For this review, take the finished solid that the model builds, in its own axes (mm). A direction names the side the tool comes from. Give positions to 0.01 mm unless a question says otherwise; leave off trailing zeros. Loops run counter-clockwise (first coordinate to the right, second up) from the corner with the lowest first, then second, coordinate; pieces in that order, holes last. Notation, with made-up numbers: (27.25, 60.25) - (68.25, 60.25) arc R23 cw to (68.25, 82.25) - close; hole circle Ø5 at (-2, -25). An arc over 180 degrees is marked (long way). Use CSV: the item, a comma, the result in double quotes. Start each with the question number.
1. Take a section at B-B on x = 0. Give the boundary of the cut face in (y, z).
2. For pin 1 (1.4 mm diameter, centred on y = 3, z = 13.5, fed in from -X); pin 2 (1.4 mm diameter, centred on y = 2.5, z = -13.5, fed in from +X), all flat-tipped, find the tip position at first contact; note any pin that passes through.
3. Take a section at C-C on z = 0. Give the boundary of the cut face in (x, y), plus the area to 3 significant figures.
4. For faces 1 (the flat face through (-4, 2, 13)), 2 (the cylindrical face through (6.59, 2.254, 11.495)), 3 (the flat face through (9.497, 2.318, -10.102)), 4 (the flat face through (-13.51, 2.32, 3.18)), list the 3-axis set-ups (+Z, -Z, +X, -X, +Y, -Y) from which the entire face can be reached by the end or side of a thin tool; tool diameter is ignored.
5. Wall thickness on line 1 (Z direction, x = 0, y = 3.6); line 2 (X direction, y = 1.9, z = 0); line 3 (Z direction, x = -8.5, y = 2.7): over which ranges is each line inside the solid? List them lowest first.
6. Mouldability with a two-part tool opening along Z and no side actions: class faces 5 (the cylindrical face through (-6.59, 2.254, -11.495)), 6 (the flat face through (-13.497, 2.318, -3.174)), 7 (the flat face through (-4, 2, -13)) as pulls with the +Z half, pulls with the -Z half, needs draft (parallel to the pull), parting line crosses it, or undercut.
7. Take a section at A-A on y = 3.75. Give the boundary of the cut face in (x, z).
```python
from build123d import *

# Parameters (mm, degrees)
SKETCH1_R           = 13.25
SKETCH1_R_2         = 10
BOSS_EXTRUDE1_DEPTH = 4.572
BOSS_EXTRUDE2_DEPTH = 4.572
CIRPATTERN1_COUNT   = 6


with BuildPart() as part:
    # Sketch1 → Boss-Extrude1 (new body)
    with BuildSketch(Plane(origin=(0, 0, 0), x_dir=(1, 0, 0), z_dir=(0, 1, 0))):
        Circle(SKETCH1_R)
        Circle(SKETCH1_R_2, mode=Mode.SUBTRACT)
    extrude(amount=BOSS_EXTRUDE1_DEPTH)

    # Sketch2 → Boss-Extrude2 (add)
    with BuildSketch(Plane(origin=(0, 4.572, 0), x_dir=(1, 0, 0), z_dir=(0, 1, 0))):
        with BuildLine():
            Line((-4, 12.631805097), (-4, 13.937359865))
            ThreePointArc((-4, 13.937359865), (0, 14.5), (4, 13.937359865))
            Line((4, 13.937359865), (4, 12.631805097))
            ThreePointArc((4, 12.631805097), (0, 13.25), (-4, 12.631805097))
        make_face()
    boss_extrude2 = extrude(amount=-BOSS_EXTRUDE2_DEPTH)

    # CirPattern1: Boss-Extrude2 ×6 about axis
    cirpattern1_axis = Axis((0, 0, 0), (0, 1, 0))
    for i in range(1, CIRPATTERN1_COUNT):
        add(boss_extrude2.rotate(cirpattern1_axis, i * 360 / CIRPATTERN1_COUNT))


solid = part.part
```
Check result:
1,outline,"(0, -14.5) - (4.57, -14.5) - (4.57, -10) - (0, -10) - close; (0, 10) - (4.57, 10) - (4.57, 14.5) - (0, 14.5) - close"
2,pin 1,"stops at x = -4"
2,pin 2,"stops at x = 4"
3,outline,"(-13.25, 0) - (-10, 0) - (-10, 4.57) - (-13.25, 4.57) - close; (10, 0) - (13.25, 0) - (13.25, 4.57) - (10, 4.57) - close"
3,area,"29.7 mm²"
4,face 1,"+Z, -X, +Y, -Y"
4,face 2,"+Z, +Y, -Y"
4,face 3,"-Z, +Y, -Y"
4,face 4,"-X, +Y, -Y"
5,line 1,"z = -14.5 to -10, 10 to 14.5"
5,line 2,"x = -13.25 to -10, 10 to 13.25"
5,line 3,"z = -10.16 to -5.27, 5.27 to 10.16"
6,face 5,"pulls with the -Z half"
6,face 6,"undercut"
6,face 7,"needs draft"
7,outline,"(-14.07, -3.5) arc R14.5 ccw to (-10.07, -10.43) - (-8.94, -9.78) arc R13.25 ccw to (-4, -12.63) - (-4, -13.94) arc R14.5 ccw to (4, -13.94) - (4, -12.63) arc R13.25 ccw to (8.94, -9.78) - (10.07, -10.43) arc R14.5 ccw to (14.07, -3.5) - (12.94, -2.85) arc R13.25 ccw to (12.94, 2.85) - (14.07, 3.5) arc R14.5 ccw to (10.07, 10.43) - (8.94, 9.78) arc R13.25 ccw to (4, 12.63) - (4, 13.94) arc R14.5 ccw to (-4, 13.94) - (-4, 12.63) arc R13.25 ccw to (-8.94, 9.78) - (-10.07, 10.43) arc R14.5 ccw to (-14.07, 3.5) - (-12.94, 2.85) arc R13.25 ccw to (-12.94, -2.85) - close; hole circle Ø20 at (0, 0)"
